Design review of the part shown in the three views and the two pictorial views. Dimensions are in mm from the part's minimum x, y and z. A direction names the side the tool comes from. Coordinates: 2 decimals unless noted, no trailing zeros. Order: outer loops, then holes, each group sorted by start corner. A loop starts at its lowest first (then second) coordinate and runs counter-clockwise, first axis right, second up. Notation, with made-up numbers: (14.5, 15) - (61.5, 15) arc R9 cw to (61.5, 20) - close; hole circle Ø5 at (3.5, 81). An arc over 180 degrees is marked (long way). One line per item, written item: value. Start each with the question number.
(1) Consider section B-B on y = 5. Write out the cut boundary in (x, z), then the cut area to 3 significant figures.
(2) Mouldability with a two-part tool opening along Y and no side actions: class the marked faces 1, 2 and 3 as released by +Y, released by -Y, zero draft, split by the parting line, or undercut.
(3) To check wall thickness, follow line 1 along Y through (x, z) = (3.5, 1.75); line 2 along Z through (x, y) = (3.5, 13.1); line 3 along Y through (x, z) = (0.5, 9). State the ranges of each line that lie inside material, in increasing order.
(4) Consider section D-D on z = 11. Write out the cut boundary in (x, y), then the cut area to 3 significant figures.
(5) Consider section C-C on y = 14. Write out the cut boundary in (x, z), then the cut area to 3 significant figures.
(6) Consider section A-A on x = 3.5. Write out the cut boundary in (y, z).
(7) For the marked faces 4 and 5, list the 3-axis set-ups (+Z, -Z, +X, -X, +Y, -Y) from which the entire face can be reached by the end or side of a thin tool; tool diameter is ignored.
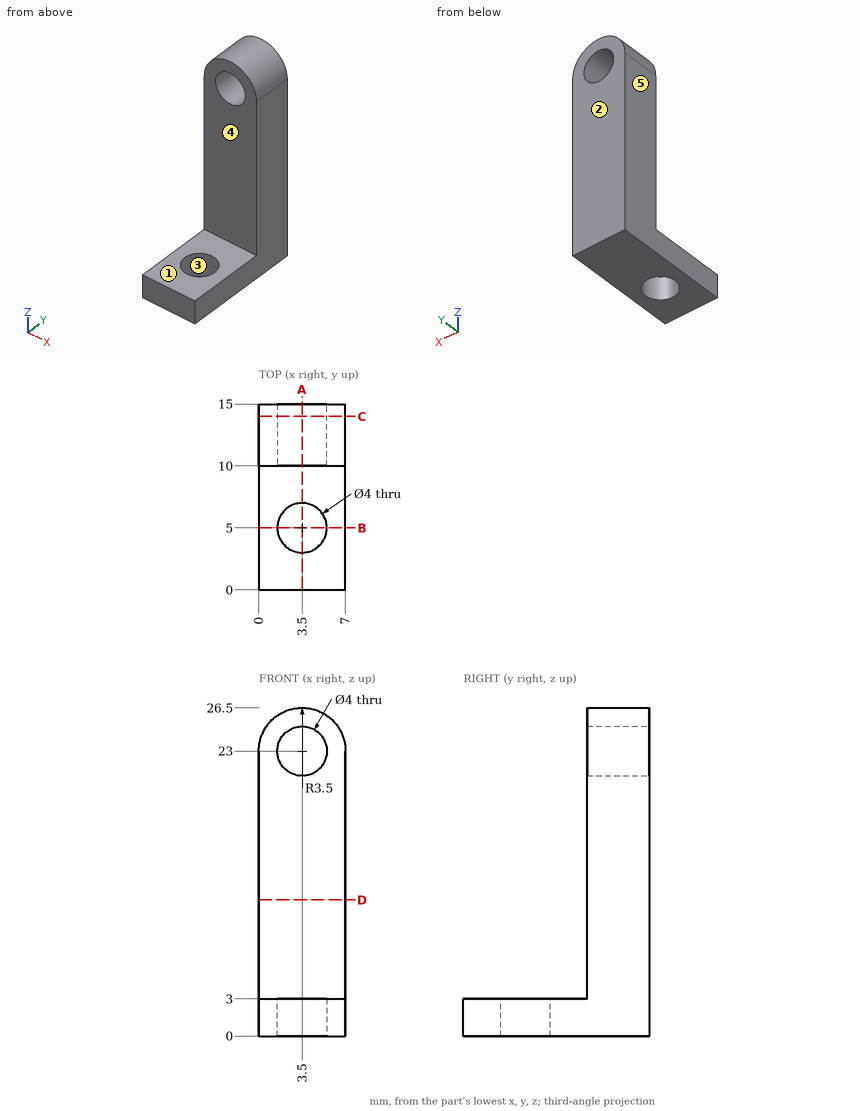
Geometry check:
1. outline: (0, 0) - (1.5, 0) - (1.5, 3) - (0, 3) - close; (5.5, 0) - (7, 0) - (7, 3) - (5.5, 3) - close
1. area: 9.00 mm^2
2. face 1: zero draft
2. face 2: released by +Y
2. face 3: undercut
3. line 1: y = 0 to 3, 7 to 15
3. line 2: z = 0 to 21, 25 to 26.5
3. line 3: y = 10 to 15
4. outline: (0, 10) - (7, 10) - (7, 15) - (0, 15) - close
4. area: 35.0 mm^2
5. outline: (0, 0) - (7, 0) - (7, 23) arc R3.5 ccw to (0, 23) - close; hole circle Ø4 at (3.5, 23)
5. area: 168 mm^2
6. outline: (0, 0) - (3, 0) - (3, 3) - (0, 3) - close; (7, 0) - (15, 0) - (15, 21) - (10, 21) - (10, 3) - (7, 3) - close; (10, 25) - (15, 25) - (15, 26.5) - (10, 26.5) - close
7. face 4: +Z, +X, -X, -Y
7. face 5: +Z, -Z, -X, +Y, -Y
